```python
from build123d import *

# Parameters (mm, degrees)
BOSS_EXTRUDE1_DEPTH = 4
BOSS_EXTRUDE1_DRAFT = 10
CUT_EXTRUDE1_START  = 4
SKETCH1_3_R         = 1.1
CUT_EXTRUDE1_DEPTH  = 4
CUT_EXTRUDE2_START  = 4
SKETCH1_4_R         = 8.4
SKETCH1_4_R_2       = 1.1
CUT_EXTRUDE2_DEPTH  = 3


# Read off the part's stored shape, not the designer's step: Boss-Extrude1
with BuildPart() as part:
    # Boss-Extrude1 outline → Boss-Extrude1 (with draft: the straight prism first)
    with BuildSketch(Plane(origin=(0, 4, 0), x_dir=(1, 0, 0), z_dir=(0, 1, 0))):
        with BuildLine():
            ThreePointArc((-78.561875024, -11.799956956), (-78.561875024, -22.494649034), (-69.3, -27.841995072))
            Line((-69.3, -27.841995072), (-9.9, -27.841995072))
            ThreePointArc((-9.9, -27.841995072), (-4.552653961, -26.409178019), (-0.638124976, -22.494649034))
            Line((-0.638124976, -22.494649034), (9.261875024, -5.347346039))
            ThreePointArc((9.261875024, -5.347346039), (9.261875024, 5.347346039), (0, 10.694692077))
            Line((0, 10.694692077), (-59.4, 10.694692077))
            ThreePointArc((-59.4, 10.694692077), (-64.747346039, 9.261875024), (-68.661875024, 5.347346039))
            Line((-68.661875024, 5.347346039), (-78.561875024, -11.799956956))
        make_face()
    extrude(amount=-BOSS_EXTRUDE1_DEPTH)
    # Boss-Extrude1: the draft: its side faces are tilted about the plane it starts from
    boss_extrude1_sides = [part.faces().sort_by_distance(p)[0] for p in [
        (-73.611875024, 2, 3.226305459),
        (-78.561875024, 2, 22.494649033),
        (-39.6, 2, 27.841995072),
        (-4.552653962, 2, 26.409178019),
        (4.311875024, 2, 13.920997536),
        (9.261875024, 2, -5.347346038),
        (-29.7, 2, -10.694692077),
        (-64.747346038, 2, -9.261875024),
    ]]
    draft(boss_extrude1_sides, Plane(origin=(0, 4, 0), x_dir=(1, 0, 0), z_dir=(0, 1, 0)), BOSS_EXTRUDE1_DRAFT)

    # Sketch1<3> → Cut-Extrude1 (cut)
    with BuildSketch(Plane(origin=(0, 0, 0), x_dir=(1, 0, 0), z_dir=(0, 1, 0)).offset(CUT_EXTRUDE1_START)):
        with Locations(Location((-9.9, -17.147302995, 0), (0, 0, 270))):
            Circle(SKETCH1_3_R)
        with Locations(Location((0, 0, 0), (0, 0, 270))):
            Circle(SKETCH1_3_R)
        with Locations(Location((-29.7, -17.147302995, 0), (0, 0, 270))):
            Circle(SKETCH1_3_R)
        with Locations(Location((-39.6, 0, 0), (0, 0, 270))):
            Circle(SKETCH1_3_R)
        with Locations(Location((-49.5, -17.147302995, 0), (0, 0, 270))):
            Circle(SKETCH1_3_R)
        with Locations(Location((-59.4, 0, 0), (0, 0, 270))):
            Circle(SKETCH1_3_R)
        with Locations(Location((-69.3, -17.147302995, 0), (0, 0, 270))):
            Circle(SKETCH1_3_R)
        with Locations(Location((-19.8, 0, 0), (0, 0, 270))):
            Circle(SKETCH1_3_R)
    extrude(amount=-CUT_EXTRUDE1_DEPTH, mode=Mode.SUBTRACT)

    # Sketch1<4> → Cut-Extrude2 (cut)
    # profile 1 of 8: a face of its own
    with BuildSketch(Plane(origin=(0, 0, 0), x_dir=(1, 0, 0), z_dir=(0, 1, 0)).offset(CUT_EXTRUDE2_START)):
        with Locations(Location((-19.8, 0, 0), (0, 0, 270))):
            Circle(SKETCH1_4_R)
        with Locations(Location((-19.8, 0, 0), (0, 0, 270))):
            Circle(SKETCH1_4_R_2, mode=Mode.SUBTRACT)
    # profile 2 of 8: a face of its own
    with BuildSketch(Plane(origin=(0, 0, 0), x_dir=(1, 0, 0), z_dir=(0, 1, 0)).offset(CUT_EXTRUDE2_START)):
        with Locations(Location((-9.9, -17.147302995, 0), (0, 0, 270))):
            Circle(SKETCH1_4_R)
        with Locations(Location((-9.9, -17.147302995, 0), (0, 0, 270))):
            Circle(SKETCH1_4_R_2, mode=Mode.SUBTRACT)
    # profile 3 of 8: a face of its own
    with BuildSketch(Plane(origin=(0, 0, 0), x_dir=(1, 0, 0), z_dir=(0, 1, 0)).offset(CUT_EXTRUDE2_START)):
        with Locations(Location((0, 0, 0), (0, 0, 270))):
            Circle(SKETCH1_4_R)
        with Locations(Location((0, 0, 0), (0, 0, 270))):
            Circle(SKETCH1_4_R_2, mode=Mode.SUBTRACT)
    # profile 4 of 8: a face of its own
    with BuildSketch(Plane(origin=(0, 0, 0), x_dir=(1, 0, 0), z_dir=(0, 1, 0)).offset(CUT_EXTRUDE2_START)):
        with Locations(Location((-29.7, -17.147302995, 0), (0, 0, 270))):
            Circle(SKETCH1_4_R)
        with Locations(Location((-29.7, -17.147302995, 0), (0, 0, 270))):
            Circle(SKETCH1_4_R_2, mode=Mode.SUBTRACT)
    # profile 5 of 8: a face of its own
    with BuildSketch(Plane(origin=(0, 0, 0), x_dir=(1, 0, 0), z_dir=(0, 1, 0)).offset(CUT_EXTRUDE2_START)):
        with Locations(Location((-39.6, 0, 0), (0, 0, 270))):
            Circle(SKETCH1_4_R)
        with Locations(Location((-39.6, 0, 0), (0, 0, 270))):
            Circle(SKETCH1_4_R_2, mode=Mode.SUBTRACT)
    # profile 6 of 8: a face of its own
    with BuildSketch(Plane(origin=(0, 0, 0), x_dir=(1, 0, 0), z_dir=(0, 1, 0)).offset(CUT_EXTRUDE2_START)):
        with Locations(Location((-49.5, -17.147302995, 0), (0, 0, 270))):
            Circle(SKETCH1_4_R)
        with Locations(Location((-49.5, -17.147302995, 0), (0, 0, 270))):
            Circle(SKETCH1_4_R_2, mode=Mode.SUBTRACT)
    # profile 7 of 8: a face of its own
    with BuildSketch(Plane(origin=(0, 0, 0), x_dir=(1, 0, 0), z_dir=(0, 1, 0)).offset(CUT_EXTRUDE2_START)):
        with Locations(Location((-59.4, 0, 0), (0, 0, 270))):
            Circle(SKETCH1_4_R)
        with Locations(Location((-59.4, 0, 0), (0, 0, 270))):
            Circle(SKETCH1_4_R_2, mode=Mode.SUBTRACT)
    # profile 8 of 8: a face of its own
    with BuildSketch(Plane(origin=(0, 0, 0), x_dir=(1, 0, 0), z_dir=(0, 1, 0)).offset(CUT_EXTRUDE2_START)):
        with Locations(Location((-69.3, -17.147302995, 0), (0, 0, 270))):
            Circle(SKETCH1_4_R)
        with Locations(Location((-69.3, -17.147302995, 0), (0, 0, 270))):
            Circle(SKETCH1_4_R_2, mode=Mode.SUBTRACT)
    extrude(amount=-CUT_EXTRUDE2_DEPTH, mode=Mode.SUBTRACT)


solid = part.part
```
The listing builds one solid part. Answer for the finished solid, in the listing's coordinates (mm). A direction names the side the tool comes from. Coordinates: 2 decimals unless noted, no trailing zeros. Loops run counter-clockwise (first coordinate to the right, second up) from the corner with the lowest first, then second, coordinate; pieces in that order, holes last. Notation, with made-up numbers: (3, 48) -> (60, 48) arc R16 ccw to (60, 55) -> close; hole circle Ø10 at (-20, -27.5). An arc over 180 degrees is marked (long way). Use one line per item in the form item = value. Start each with the question number.
Item 1: The mould has two halves that part along Z. Classify faces 3 (the face through (-64.851, 2.028, -9.603)), 4 (the face through (-60.97, 2.52, 16.05)), 5 (the face through (-35, 4, 8)), 6 (the face through (1.09, 0.51, -0.14)): released by +Z, released by -Z, zero draft, split by the parting line, or undercut.
Item 2: Flat-ended cylindrical pins translate along their axes: pin 1 Ø5 at (x, z) = (-30.5, 17) entering from +Y; pin 2 Ø1 at (y, z) = (2.5, 4.5) entering from +X; pin 3 Ø1 at (y, z) = (1.5, 7) entering from +X. Find the tip coordinate at first contact, or state that the pin passes through.
Item 3: Consider L1, parallel to X at y = 3.05, z = -7; L2, parallel to X at y = 2.45, z = -5.5; L3, parallel to Z at x = -6, y = 1.8. Determine where each line is inside the solid, lowest interval first. Write a range as [from, to].
Item 4: The part is cut by section C-C on x = -17. Determine the outline of the cut face in (y, z), then the cut area to 3 significant figures.
Item 5: A tool of negligible diameter and unlimited length cuts with its end or side. For faces 1 (the face through (-35, 0, 8)), 2 (the face through (-22, 1, 0)), from which of +Z, -Z, +X, -X, +Y, -Y can it reach the whole face along a straight path? Write none if from no direction.
Item 6: The part is cut by section D-D on x = -53.5. Determine the outline of the cut face in (y, z).
Item 7: The part is cut by section A-A on x = -39.6. Determine the outline of the cut face in (y, z).
Item 8: The part is cut by section B-B on y = 2.75. Count the separate pieces of the cut face and the enclosed holes in it, then the cut area to 3 significant figures.
Answer key:
q1.face_3 = released by -Z
q1.face_4 = undercut
q1.face_5 = zero draft
q1.face_6 = undercut
q2.pin_1 = 1
q2.pin_2 = 10.22
q2.pin_3 = 9.12
q3.L1 = [-67.71, -64.04], [-54.76, -44.24], [-34.96, -24.44], [-15.16, -4.64], [4.64, 8.31]
q3.L2 = [-68.89, -65.75], [-53.05, -45.95], [-33.25, -26.15], [-13.45, -6.35], [6.35, 9.49]
q3.L3 = [-11.08, -5.88], [5.88, 9.71], [24.59, 27.52]
q4.outline = (0, -11.4) -> (4, -10.69) -> (4, -7.92) -> (1, -7.92) -> (1, 7.92) -> (4, 7.92) -> (4, 12.66) -> (1, 12.66) -> (1, 21.64) -> (4, 21.64) -> (4, 27.84) -> (0, 28.55) -> close
q4.area = 82.5 mm2
q5.face_1 = +Z, -Z, +X, -X, -Y
q5.face_2 = +Y
q6.outline = (0, -11.4) -> (4, -10.69) -> (4, -5.98) -> (1, -5.98) -> (1, 5.98) -> (4, 5.98) -> (4, 9.76) -> (1, 9.76) -> (1, 24.53) -> (4, 24.53) -> (4, 27.84) -> (0, 28.55) -> close
q7.outline = (0, -11.4) -> (4, -10.69) -> (4, -8.4) -> (1, -8.4) -> (1, -1.1) -> (0, -1.1) -> close; (0, 1.1) -> (1, 1.1) -> (1, 8.4) -> (4, 8.4) -> (4, 27.84) -> (0, 28.55) -> close
q8.separate_pieces = 1
q8.enclosed_holes = 8
q8.area = 1,350 mm2
